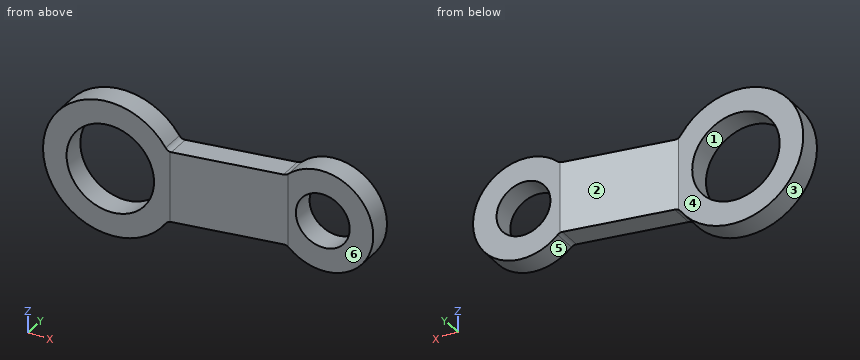
from build123d import *

# Parameters (mm, degrees)
F0_R     = 33.02
F0_R_2   = 20.32
F1_DEPTH = 50.8
F3_DEPTH = 50.8
F4_R     = 5.08
F5_R     = 5.08
F6_R     = 5.08
F7_R     = 5.08


with BuildPart() as f1:
    # F0 (on Front) → F1 (new body)
    with BuildSketch(Plane.XZ):
        with BuildLine():
            ThreePointArc((43.2359931076, -26.67), (48.8724280646, -13.8609442343), (50.8, 0))
            ThreePointArc((50.8, 0), (48.8724280646, 13.8609442343), (43.2359931076, 26.67))
            ThreePointArc((43.2359931076, 26.67), (-50.8, 0), (43.2359931076, -26.67))
        make_face()
        Circle(F0_R, mode=Mode.SUBTRACT)
        with BuildLine():
            ThreePointArc((43.2359931076, 26.67), (48.8724280646, 13.8609442343), (50.8, 0))
            ThreePointArc((50.8, 0), (48.8724280646, -13.8609442343), (43.2359931076, -26.67))
            Line((43.2359931076, -26.67), (125.1911576873, -26.67))
            ThreePointArc((125.1911576873, -26.67), (114.3, 0), (125.1911576873, 26.67))
            Line((125.1911576873, 26.67), (43.2359931076, 26.67))
        make_face()
        with BuildLine():
            ThreePointArc((190.5, 0), (166.8040464433, 35.2722758843), (125.1911576873, 26.67))
            ThreePointArc((125.1911576873, 26.67), (114.3, 0), (125.1911576873, -26.67))
            ThreePointArc((125.1911576873, -26.67), (166.8040464433, -35.2722758843), (190.5, 0))
        make_face()
        with Locations((152.4, 0)):
            Circle(F0_R_2, mode=Mode.SUBTRACT)
    extrude(amount=F1_DEPTH)

    # F2 (on Top) → F3 (intersect, symmetric)
    with BuildSketch(Plane.XY):
        Polygon((213.7089745641, -17.78), (213.7089745641, 0), (124.8089745641, 0), (43.4407666326, -13.5890487581), (-83.5592333674, -13.5890487581), (-83.5592333674, -31.3690487581), (44.915247018, -31.3690487581), (126.2834549495, -17.78), align=None)
    extrude(amount=F3_DEPTH, both=True, mode=Mode.INTERSECT)

    # F4
    f4_edges = [f1.edges().sort_by_distance(p)[0] for p in [
        (43.235993, -22.479049, 26.67),
    ]]
    fillet(f4_edges, radius=F4_R)

    # F5
    f5_edges = [f1.edges().sort_by_distance(p)[0] for p in [
        (125.191158, -8.981211, 26.67),
    ]]
    fillet(f5_edges, radius=F5_R)

    # F6
    f6_edges = [f1.edges().sort_by_distance(p)[0] for p in [
        (43.235993, -22.479049, -26.67),
    ]]
    fillet(f6_edges, radius=F6_R)

    # F7
    f7_edges = [f1.edges().sort_by_distance(p)[0] for p in [
        (125.191158, -8.981211, -26.67),
    ]]
    fillet(f7_edges, radius=F7_R)


solid = f1.part
Could you check a few things on this model? Use its own coordinates, in mm. Face numbers are marked on the shaded views. A direction names the side the tool comes from. Give positions to 0.01 mm unless a question says otherwise; leave off trailing zeros. Order: outer loops, then holes, each group sorted by start corner. A loop starts at its lowest first (then second) coordinate and runs counter-clockwise, first axis right, second up. Notation, with made-up numbers: (-26, -8.75) -> (-11, -8.75) arc R23 cw to (-11, 21.25) -> close; hole circle Ø9 at (56.25, 54). An arc over 180 degrees is marked (long way). Return JSON: item names as keys, results as strings.
1. Imagine slicing it at A-A on x = 0. List the corners of the cut face in (y, z) for me.
Answer list:
{"outline": "(-31.37, -50.8) -> (-13.59, -50.8) -> (-13.59, -33.02) -> (-31.37, -33.02) -> close; (-31.37, 33.02) -> (-13.59, 33.02) -> (-13.59, 50.8) -> (-31.37, 50.8) -> close"}
2. For pin 1 Ø5 at (y, z) = (-22.5, -9.5) entering from -X; pin 2 Ø19.5 at (x, z) = (161, -16.5) entering from -Y; pin 3 Ø9.5 at (x, y) = (79, -8.5) entering from -Z, each with a flat end and sliding along its axis, tell me the tip position at first contact or that it passes through.
Answer list:
{"pin 1": "stops at x = -50.32", "pin 2": "stops at y = -17.78", "pin 3": "stops at z = -26.67"}
3. I need wall thicknesses on line 1 (Z direction, x = 0, y = -18.5); line 2 (Z direction, x = 152.4, y = -7.5); line 3 (Y direction, x = 28, z = 41.5). Which ranges of each line are inside material? Lowest first, please. Write a range as from..to.
Answer list:
{"line 1": "z = -50.8..-33.02, 33.02..50.8", "line 2": "z = -38.1..-20.32, 20.32..38.1", "line 3": "y = -31.37..-13.59"}
4. On a 3-axis mill with a long thin cutter (end or side, diameter ignored), from which of +Z, -Z, +X, -X, +Y, -Y can I reach the whole of each face in a straight line? I mean the marked faces 4, 5 and 6. Say none if no direction works.
Answer list:
{"face 4": "+Z, -Z, -X, +Y", "face 5": "+Y, -Y", "face 6": "+Z, -Z, +X, -Y"}
5. Thinking about a two-plate mould opening in Z: for the marked faces 1, 2 and 3, which applies, pulls with the +Z half, pulls with the -Z half, needs draft (parallel to the pull), parting line crosses it, or undercut?
Answer list:
{"face 1": "undercut", "face 2": "needs draft", "face 3": "parting line crosses it"}
6. Imagine slicing it at B-B on z = 0. List the corners of the cut face in (x, y) for me, then the cut area to 3 significant figures.
Answer list:
{"outline": "(-50.8, -31.37) -> (-33.02, -31.37) -> (-33.02, -13.59) -> (-50.8, -13.59) -> close; (33.02, -31.37) -> (44.92, -31.37) -> (126.28, -17.78) -> (132.08, -17.78) -> (132.08, 0) -> (124.81, 0) -> (43.44, -13.59) -> (33.02, -13.59) -> close; (172.72, -17.78) -> (190.5, -17.78) -> (190.5, 0) -> (172.72, 0) -> close", "area": "2,410 mm2"}
7. Imagine slicing it at D-D on z = 17. List the corners of the cut face in (x, y) for me, then the cut area to 3 significant figures.
Answer list:
{"outline": "(-47.87, -31.37) -> (-28.31, -31.37) -> (-28.31, -13.59) -> (-47.87, -13.59) -> close; (28.31, -31.37) -> (44.92, -31.37) -> (126.28, -17.78) -> (141.27, -17.78) -> (141.27, 0) -> (124.81, 0) -> (43.44, -13.59) -> (28.31, -13.59) -> close; (163.53, -17.78) -> (186.5, -17.78) -> (186.5, 0) -> (163.53, 0) -> close", "area": "2,780 mm2"}
8. Imagine slicing it at C-C on y = -29. List the corners of the cut face in (x, z) for me, then the cut area to 3 significant figures.
Answer list:
{"outline": "(41.8, -28.86) arc R5.08 cw to (45.98, -26.67) -> (59.1, -26.67) -> (59.1, 26.67) -> (45.98, 26.67) arc R5.08 cw to (41.8, 28.86) arc R50.8 ccw (long way) to start; hole circle Ø66.04 at (0, 0)", "area": "5,260 mm2"}
